Geometry check sheet. Reference: drawing and pictorial views, mm from the part's lowest x, y, z. Round coordinates to 2 decimals unless told otherwise and drop trailing zeros. Write each loop counter-clockwise with the first axis right and the second up, starting at its lowest first coordinate (ties: lowest second). Pieces come first, ordered by that corner, then holes. Notation, with made-up numbers: M 83,-31.5 L 93,-31.5 A32 cw 93,-0.5 Z; hole C -16,-13 d11. An arc over 180 degrees is marked long. Answer in a Markdown table with one row per item. Add a question column.
1. Material ranges on probe 1 along Y at (x, z) = (22, 11); probe 2 along Y at (x, z) = (148, 18.25); probe 3 along X at (y, z) = (194.5, 15), recorded low to high.
2. Sectioned sample at D-D on x = 98. Record the cut outline in (y, z), plus the area to 3 significant figures.
3. Sectioned sample at A-A on y = 46. Record the cut outline in (x, z), plus the area to 3 significant figures.
4. Sectioned sample at B-B on x = 148. Record the cut outline in (y, z), plus the area to 3 significant figures.
5. Draft check along Y on the marked faces 1, 2, 3 and 4. Enter one of: pulls with the +Y half, pulls with the -Y half, needs draft (parallel to the pull), parting line crosses it, or undercut.
6. Sectioned sample at C-C on z = 14.75. Count the separate pieces of the cut face and the enclosed holes in it, plus the area to 3 significant figures.
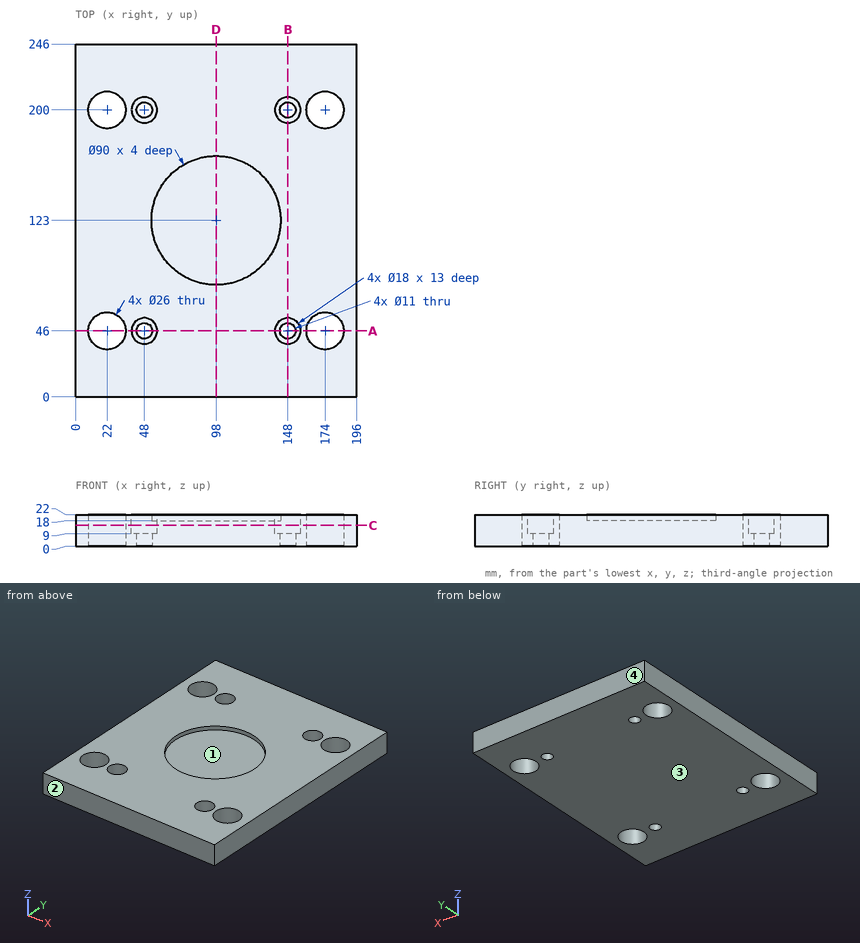
Geometry check:
| question | item | result |
|---|---|---|
| 1 | probe 1 | y = 0 to 33, 59 to 187, 213 to 246 |
| 1 | probe 2 | y = 0 to 37, 55 to 191, 209 to 246 |
| 1 | probe 3 | x = 0 to 10.22, 33.78 to 40.88, 55.12 to 140.88, 155.12 to 162.22, 185.78 to 196 |
| 2 | outline | M 0,0 L 246,0 L 246,22 L 168,22 L 168,18 L 78,18 L 78,22 L 0,22 Z |
| 2 | area | 5,050 mm2 |
| 3 | outline | M 0,0 L 9,0 L 9,22 L 0,22 Z; M 35,0 L 42.5,0 L 42.5,9 L 39,9 L 39,22 L 35,22 Z; M 53.5,0 L 142.5,0 L 142.5,9 L 139,9 L 139,22 L 57,22 L 57,9 L 53.5,9 Z; M 153.5,0 L 161,0 L 161,22 L 157,22 L 157,9 L 153.5,9 Z; M 187,0 L 196,0 L 196,22 L 187,22 Z |
| 3 | area | 2,500 mm2 |
| 4 | outline | M 0,0 L 40.5,0 L 40.5,9 L 37,9 L 37,22 L 0,22 Z; M 51.5,0 L 194.5,0 L 194.5,9 L 191,9 L 191,22 L 55,22 L 55,9 L 51.5,9 Z; M 205.5,0 L 246,0 L 246,22 L 209,22 L 209,9 L 205.5,9 Z |
| 4 | area | 4,750 mm2 |
| 5 | face 1 | undercut |
| 5 | face 2 | pulls with the -Y half |
| 5 | face 3 | needs draft |
| 5 | face 4 | pulls with the +Y half |
| 6 | separate pieces | 1 |
| 6 | enclosed holes | 8 |
| 6 | area | 45,100 mm2 |
